The listing builds one solid part. Answer for the finished solid, in the listing's coordinates (mm). Face numbers are marked on the shaded views. Give positions to 0.01 mm unless a question says otherwise; leave off trailing zeros. Order: outer loops, then holes, each group sorted by start corner. A loop starts at its lowest first (then second) coordinate and runs counter-clockwise, first axis right, second up. Notation, with made-up numbers: (65, 61.25) - (101, 61.25) arc R20 ccw to (101, 71.25) - close; hole circle Ø2 at (54, -30). An arc over 180 degrees is marked (long way). Answer in a Markdown table with one row per item. Add a question column.
Solid Edge part; units mm, degrees
sketch "Sketch1" plane through (0, 0, 0) normal (0, 0, 1) x (1, 0, 0)
  circle A0 centre (-71.6995, 49.2327) radius 50
extrude "Protrusion1" add sketch "Sketch1" along normal blind 55
sketch "Sketch2" plane through (-71.6995, 49.2327, 55) normal (0, 0, 1) x (1, 0, 0)
  circle A0 centre (0, 0) radius 30
extrude "ExtrudedCutout_1" cut sketch "Sketch2" against normal blind 50
sketch "Sketch3" plane through (-71.6995, 0, 0) normal (1, 0, 0) x (0, 1, 0)
  line L0 (99.2327, 0) -> (49.2327, 0)
  arc A0 (53.3155, -32.8588) -> (49.2327, -30) centre (49.2327, -34.3448) ccw
  arc A1 (53.3155, -32.8588) -> (70.6979, -9.5837) centre (73.0225, -29.4481) cw
  line L1 (70.6979, -9.5837) -> (99.2327, 0)
  dimension "D1" = 99.2327
revolve "RevolvedProtrusion1" add sketch "Sketch3" angle 360 about axis through (-71.6995, 49.2327, 0) along (0, 0, -1)
properties material "Aluminum, 6061-T6"
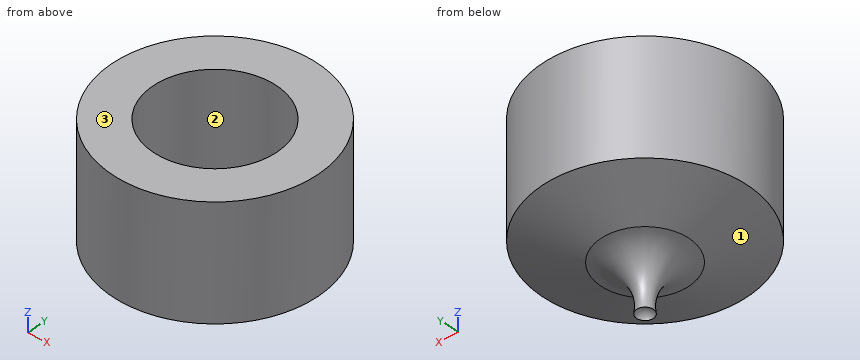
(1) The mould has two halves that part along Y. Classify the marked faces 1, 2 and 3: +Y half, -Y half, draft (parallel to the pull), parting line (faces both ways), or undercut.
(2) Straight lines are drawn through the part: line 1 (Y direction, x = -70.5, z = 49); line 2 (Y direction, x = -71, z = 10); line 3 (X direction, y = 56.5, z = 16). For each, find the intervals that lie inside material, in ascending order.
(3) Find section A-A, the plane z = 46. Write down the section's boundary in (x, y), plus the area to 3 significant figures.
(4) Find section C-C, the plane z = -2. Write down the section's boundary in (x, y).
(5) Each of these flat-tipped pins is pushed along its axis until it touches: P1, Ø2, axis at y = 31, z = 16.5, coming from the -X side; P2, Ø3, axis at y = 87.5, z = 28.5, coming from the -X side; P3, Ø6, axis at y = 43.5, z = -17, coming from the +X side. Where does it stop, or does it pass through?
(6) Find section B-B, the plane z = -22.5. Write down the section's boundary in (x, y), plus the area to 3 significant figures.
Answer key:
| question | item | result |
|---|---|---|
| 1 | face 1 | parting line |
| 1 | face 2 | undercut |
| 1 | face 3 | draft |
| 2 | line 1 | -0.75 to 19.26, 79.21 to 99.22 |
| 2 | line 2 | -0.76 to 19.24, 79.22 to 99.23 |
| 2 | line 3 | -121.17 to -100.81, -42.59 to -22.23 |
| 3 | outline | circle Ø100 at (-71.7, 49.23); hole circle Ø60 at (-71.7, 49.23) |
| 3 | area | 5,030 mm² |
| 4 | outline | circle Ø88.09 at (-71.7, 49.23) |
| 5 | P1 | x = -118.64 |
| 5 | P2 | x = -105.58 |
| 5 | P3 | x = -61.9 |
| 6 | outline | circle Ø10.07 at (-71.7, 49.23) |
| 6 | area | 79.7 mm² |
